Geometry: final body of the model. Coordinates: model frame, mm. Give positions to 0.01 mm unless a question says otherwise; leave off trailing zeros. Order: outer loops, then holes, each group sorted by start corner. A loop starts at its lowest first (then second) coordinate and runs counter-clockwise, first axis right, second up. Notation, with made-up numbers: M -33,50 L 21,50 A16 cw 21,81 Z; hole C 51,19.5 d8. An arc over 180 degrees is marked long. Use CSV: the item, a comma, the result in double quotes.
Autodesk Inventor part; units mm, degrees
ref_plane "Work Plane1" through (-12.4358, 0, 0) normal (0, -0.8660254, -0.5) x (1, 0, 0)
ref_plane "YZ Plane" through (0, 0, 0) normal (1, 0, 0) x (0, 1, 0)
ref_plane "XZ Plane" through (0, 0, 0) normal (0, 1, 0) x (-1, 0, 0)
sketch "Szkic1" plane through (0, 0, 0) normal (1, 0, 0) x (0, 1, 0)
  line L0 (-5.7735, 0) -> (-2.8868, 5)
  line L1 (-2.8868, 5) -> (2.8868, 5)
  line L2 (2.8868, 5) -> (5.7735, 0)
  line L3 (5.7735, 0) -> (2.8868, -5)
  line L4 (2.8868, -5) -> (-2.8868, -5)
  line L5 (-2.8868, -5) -> (-5.7735, 0)
  point P0 (0, 0)
  point P1 (0, 0)
  dimension "d0" = 11.547
extrude "Bryła" add sketch "Szkic1" along normal blind 3.2
sketch "Szkic2" plane through (0, 0, 0) normal (0, 0, 1) x (1, 0, 0)
  line L0 (0, 2.8868) -> (0, 5.7735)
  line L1 (0, 5.7735) -> (3.2, 5.7735)
  line L2 (3.2, 2.8868) -> (3.2, 5.7735)
  line L3 (-0.64, 0) -> (3.84, 0)
  line L4 (0.7641, 5.7735) -> (0, 4.45)
  line L5 (2.4359, 5.7735) -> (3.2, 4.45)
  dimension "d3" = 30
  dimension "d4" = 30
  dimension "d5" = 8.9
  dimension "d6" = 8.9
revolve "Faza1" cut sketch "Szkic2" angle 360 about axis through (-10, 0, 0) along (1, 0, 0)
sketch "Szkic3" plane through (3.2, 0, 0) normal (1, 0, 0) x (0, 0, -1)
  arc A0 (-0.625, -1.0825) -> (0.625, -1.0825) centre (0, 0) ccw
hole "Gwint" at (3.2, 0, 0) direction (-1, 0, 0) diameter 4.917 end through all
chamfer "Faza2" distance 0.5413 angle 30 1 edges at (3.2, 0, 2.4585) measured on face at (3.2, 3.7371, -0.4538)
chamfer "Faza3" distance 0.5413 angle 30 1 edges at (0, 0, 2.4585) measured on face at (0, 3.7371, -0.4538)
ref_plane "Work Plane1" through (-12.4358, 0, 0) normal (0, -0.8660254, -0.5) x (1, 0, 0)
equation "\"d0\" = 1.1547 * SW"
equation "\"d1\" = KOH"
equation "\"d3\" = ANG1"
equation "\"d4\" = ANG2"
equation "\"d5\" = SW0"
equation "\"d6\" = SW01"
equation "\"d8\" = -0.5 * GD1 + 0.5 * NND"
equation "\"d40\" = -0.5 * GD1 + 0.5 * NND"
equation "\"d10\" = -0.5 * GD1 + 0.5 * NND"
equation "\"d41\" = -0.5 * GD1 + 0.5 * NND"
equation "\"ANG1\" = 30deg"
equation "\"ANG2\" = 30deg"
equation "\"NND\" = 6"
equation "\"KOH\" = 3.2"
equation "\"SW0\" = 8.9"
equation "\"SW01\" = SW0"
equation "\"GUL\" = 0.541266 * PTC"
equation "\"THREADDIA\" = 6"
equation "\"TOA\" = 30deg"
equation "\"PTC\" = 1"
equation "\"E0\" = 1.155 * SW"
equation "\"GAL\" = 0.541266 * PTC"
properties part number "ISO 4035 - M6" material "Stal nierdzewna 440C"
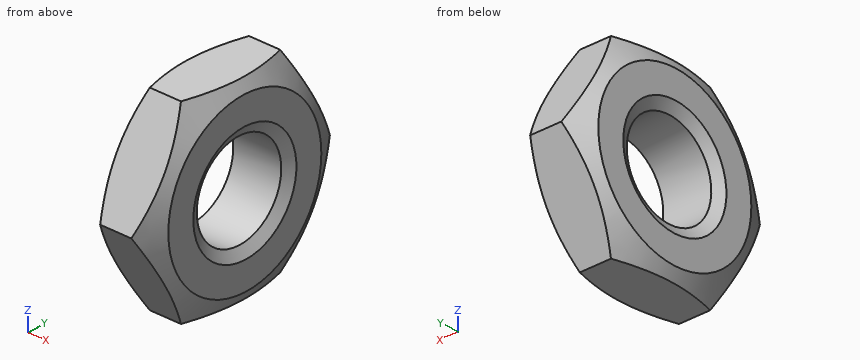
1. Line query: line 1 (Z direction, x = 1.45, y = 0); line 2 (Z direction, x = 2.1, y = -0.75). Output: solid intervals per line, ascending.
Answer:
line 1,"-5 to -2.46, 2.46 to 5"
line 2,"-5 to -2.34, 2.34 to 5"
2. Section C-C, the plane x = 1.55. Return the cut outline in (y, z), plus the area to 3 significant figures.
Answer:
outline,"M -5.77,0 L -2.89,-5 L 2.89,-5 L 5.77,0 L 2.89,5 L -2.89,5 Z; hole C 0,0 d4.92"
area,"67.6 mm2"
3. Section B-B, the plane x = 2.7. Return the cut outline in (y, z), plus the area to 3 significant figures.
Answer:
outline,"M -5.23,-0.94 L -3.43,-4.06 A5.32 ccw -1.81,-5 L 1.81,-5 A5.32 ccw 3.43,-4.06 L 5.23,-0.94 A5.32 ccw 5.23,0.94 L 3.43,4.06 A5.32 ccw 1.81,5 L -1.81,5 A5.32 ccw -3.43,4.06 L -5.23,0.94 A5.32 ccw Z; hole C 0,0 d4.92"
area,"65.2 mm2"
4. Pin query (flat end, axial travel): pin 1 Ø3 at (y, z) = (0, 0) entering from +X. Return the tip coordinate at first contact, or that it passes through.
Answer:
pin 1,"through"
5. Section A-A, the plane y = 0. Return the cut outline in (x, z), plus the area to 3 significant figures.
Answer:
outline,"M 0,-4.45 L 0.32,-5 L 2.88,-5 L 3.2,-4.45 L 3.2,-3 L 2.89,-2.46 L 0.31,-2.46 L 0,-3 Z; M 0,3 L 0.31,2.46 L 2.89,2.46 L 3.2,3 L 3.2,4.45 L 2.88,5 L 0.32,5 L 0,4.45 Z"
area,"15.6 mm2"
